from build123d import *

# Parameters (mm, degrees)
BOSS_EXTRUDE1_DEPTH = 6.1087
CUT_EXTRUDE1_DEPTH  = 30.462097676
SKETCH3_W           = 32.8422
SKETCH3_H           = 18.608676988
BOSS_EXTRUDE2_DEPTH = 3.3274


with BuildPart() as part:
    # Sketch1 → Boss-Extrude1 (new, symmetric)
    with BuildSketch(Plane.XY):
        Polygon((-27.4574, 0), (27.4574, 0), (27.4574, 2.7686), (18.0721, 2.7686), (18.0721, 11.5316), (-18.0721, 11.5316), (-18.0721, 2.7686), (-27.4574, 2.7686), align=None)
    extrude(amount=BOSS_EXTRUDE1_DEPTH, both=True)

    # Sketch2 → Cut-Extrude1 (cut, through all)
    with BuildSketch(Plane(origin=(0, 2.7686, 0), x_dir=(1, 0, 0), z_dir=(0, 1, 0))):
        with BuildLine():
            Line((-21.36775, 2.3241), (-21.36775, -2.3241))
            ThreePointArc((-21.36775, -2.3241), (-22.76475, -3.7211), (-24.16175, -2.3241))
            Line((-24.16175, -2.3241), (-24.16175, 2.3241))
            ThreePointArc((-24.16175, 2.3241), (-22.76475, 3.7211), (-21.36775, 2.3241))
        make_face()
        with BuildLine():
            Line((21.36775, 2.3241), (21.36775, -2.3241))
            ThreePointArc((21.36775, -2.3241), (22.76475, -3.7211), (24.16175, -2.3241))
            Line((24.16175, -2.3241), (24.16175, 2.3241))
            ThreePointArc((24.16175, 2.3241), (22.76475, 3.7211), (21.36775, 2.3241))
        make_face()
    extrude(amount=-CUT_EXTRUDE1_DEPTH, mode=Mode.SUBTRACT)

    # Sketch3 → Boss-Extrude2 (add)
    with BuildSketch(Plane(origin=(0, 0, -6.1087), x_dir=(-1, 0, 0), z_dir=(0, 0, -1))):
        with Locations((0, 9.304338494)):
            Rectangle(SKETCH3_W, SKETCH3_H)
    extrude(amount=BOSS_EXTRUDE2_DEPTH)


solid = part.part
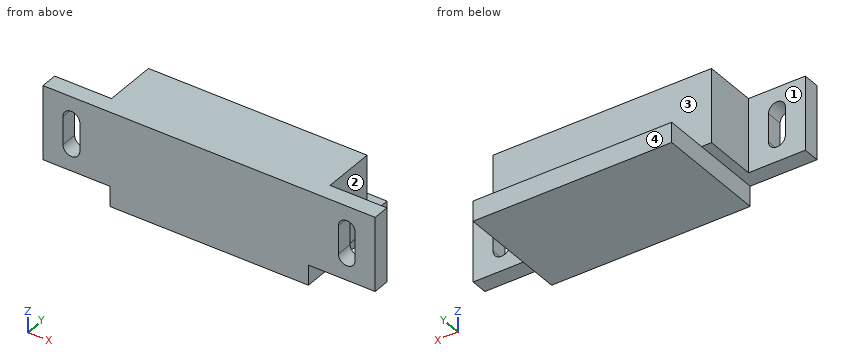
The listing builds one solid part. Answer for the finished solid, in the listing's coordinates (mm). Face numbers are marked on the shaded views. A direction names the side the tool comes from. Coordinates: 2 decimals unless noted, no trailing zeros. Write each loop counter-clockwise with the first axis right and the second up, starting at its lowest first coordinate (ties: lowest second). Pieces come first, ordered by that corner, then holes. Notation, with made-up numbers: (79.25, 24.5) - (103.25, 24.5) arc R27 ccw to (103.25, 49.5) - close; hole circle Ø3 at (74.25, 13.25). An arc over 180 degrees is marked (long way). Put each result on its own line as item: value.
1. The part is cut by section A-A on z = -1.25. Give the vertices of the cut face in (x, y), plus the area to 3 significant figures.
Answer sheet:
outline: (-27.46, 0) - (-24.16, 0) - (-24.16, 2.77) - (-27.46, 2.77) - close; (-21.37, 0) - (21.37, 0) - (21.37, 2.77) - (18.07, 2.77) - (18.07, 11.53) - (-18.07, 11.53) - (-18.07, 2.77) - (-21.37, 2.77) - close; (24.16, 0) - (27.46, 0) - (27.46, 2.77) - (24.16, 2.77) - close
area: 453 mm^2
2. The part is cut by section D-D on z = -5.5. Give the vertices of the cut face in (x, y).
Answer sheet:
outline: (-27.46, 0) - (27.46, 0) - (27.46, 2.77) - (18.07, 2.77) - (18.07, 11.53) - (-18.07, 11.53) - (-18.07, 2.77) - (-27.46, 2.77) - close
3. The part is cut by section C-C on x = 22.5. Give the vertices of the cut face in (y, z).
Answer sheet:
outline: (0, -6.11) - (2.77, -6.11) - (2.77, -3.7) - (0, -3.7) - close; (0, 3.7) - (2.77, 3.7) - (2.77, 6.11) - (0, 6.11) - close
4. Flat-ended cylindrical pins translate along their axes: pin 1 Ø2.5 at (y, z) = (8, 2.5) entering from +X; pin 2 Ø3.5 at (x, y) = (7.5, 14.5) entering from +Z; pin 3 Ø4.5 at (x, z) = (-24.5, 1.5) entering from +Y. Find the tip coordinate at first contact, or state that the pin passes through.
Answer sheet:
pin 1: stops at x = 18.07
pin 2: stops at z = -6.11
pin 3: stops at y = 2.77
5. Find the intervals of material crossed by line 1 along Z through (x, y) = (12.5, 15); line 2 along Y through (x, z) = (17.5, -0.25); line 3 along X through (y, z) = (6.25, 1), in increasing order. Write a range as from..to.
Answer sheet:
line 1: z = -9.44..-6.11
line 2: y = 0..11.53
line 3: x = -18.07..18.07
6. The part is cut by section B-B on y = 2.25. Give the vertices of the cut face in (x, z), plus the area to 3 significant figures.
Answer sheet:
outline: (-27.46, -6.11) - (-16.42, -6.11) - (-16.42, -9.44) - (16.42, -9.44) - (16.42, -6.11) - (27.46, -6.11) - (27.46, 6.11) - (-27.46, 6.11) - close; hole (-24.16, -2.32) arc R1.4 ccw to (-21.37, -2.32) - (-21.37, 2.32) arc R1.4 ccw to (-24.16, 2.32) - close; hole (21.37, -2.32) arc R1.4 ccw to (24.16, -2.32) - (24.16, 2.32) arc R1.4 ccw to (21.37, 2.32) - close
area: 742 mm^2
7. A tool of negligible diameter and unlimited length cuts with its end or side. For the marked faces 1, 2, 3 and 4, from which of +Z, -Z, +X, -X, +Y, -Y can it reach the whole face along a straight path? Write none if from no direction.
Answer sheet:
face 1: +Z, -Z, -X, +Y
face 2: +Z, -Z, +X, +Y
face 3: +Z, +X, -X, +Y
face 4: +Z, -Z, +X, -X, +Y
